The model under review builds one solid part; all positions refer to its coordinate system, in mm. A direction names the side the tool comes from. Round coordinates to 2 decimals unless told otherwise and drop trailing zeros. Write each loop counter-clockwise with the first axis right and the second up, starting at its lowest first coordinate (ties: lowest second). Pieces come first, ordered by that corner, then holes. Notation, with made-up numbers: (82, -16) -> (139, -16) arc R29 cw to (139, 4) -> close; hole circle Ø9 at (50.25, 41). An arc over 180 degrees is marked (long way). Answer as a JSON object with one key per item and string values. Group by question number.
1) Machinability: for faces 5 (the flat face through (-9.605, -0.089, 50.386)), 6 (the flat face through (-41.67, -0.09, -44.02)), 7 (the flat face through (-1, 0, 9.919)), 8 (the flat face through (101.346, 0, -27)), which of the approach directions +Z, -Z, +X, -X, +Y, -Y give a long, thin tool a straight path to every point of the face, cutting with its end or side? Answer none if there is none.
2) We need section A-A, the plane x = -20. Write out the cut boundary in (y, z).
3) We need section D-D, the plane x = 56. Write out the cut boundary in (y, z), then the cut area to 3 significant figures.
4) To check wall thickness, follow probe 1 along Z at (x, y) = (-4.5, -4.25); probe 2 along Z at (x, y) = (28, -4.75); probe 3 along X at (y, z) = (4.5, 41). State the ranges of each line that lie inside material, in increasing order. Write a range as [from, to].
5) Insertion check: pin 1 Ø2 at (x, y) = (-40, 4.5) entering from -Z; pin 2 Ø4 at (x, y) = (-4, -1.5) entering from -Z; pin 3 Ø6.5 at (x, y) = (91, -1.5) entering from +Z. Each pin has a flat end and moves straight along its axis. Give the tip position at first contact, or say it passes through.
6) We need section C-C, the plane z = -14. Write out the cut boundary in (x, y), then the cut area to 3 significant figures.
7) Mouldability with a two-part tool opening along Z and no side actions: class faces 1 (the flat face through (89, 0, -16.37)), 2 (the flat face through (-1, -6.35, -18)), 3 (the flat face through (9.697, -0.089, 50.731)), 4 (the flat face through (-75.946, 0, -7)) as pulls with the +Z half, pulls with the -Z half, needs draft (parallel to the pull), parting line crosses it, or undercut.
from build123d import *

# Parameters (mm, degrees)
F1_DEPTH = 6.35
F2_SIZE  = 12.446


with BuildPart() as f1:
    # F0 (on Front) → F1 (new body, symmetric)
    with BuildSketch(Plane.XZ):
        with BuildLine():
            Line((6.35, 38.239533), (0, 38.239533))
            Line((0, 38.239533), (-6.35, 38.239533))
            Line((-6.35, 38.239533), (-12.951732, 62.877533))
            Line((-12.951732, 62.877533), (-28.495513, 62.877533))
            ThreePointArc((-28.495513, 62.877533), (-39.577525, 59.32242), (-46.523284, 49.983992))
            ThreePointArc((-46.523284, 49.983992), (-55.553194, 36.446133), (-70.104, 29.160052))
            Line((-70.104, 29.160052), (-91.232227, 24.765415))
            ThreePointArc((-91.232227, 24.765415), (-98.498286, 20.345425), (-101.346, 12.331533))
            Line((-101.346, 12.331533), (-101.346, 2.679533))
            Line((-101.346, 2.679533), (-75.946, 2.679533))
            Line((-75.946, 2.679533), (-75.946, -16.370467))
            Line((-75.946, -16.370467), (-101.346, -16.370467))
            Line((-101.346, -16.370467), (-101.346, -50.152467))
            Line((-101.346, -50.152467), (-45.212, -50.152467))
            Line((-45.212, -50.152467), (-38.026299, -37.706467))
            Line((-38.026299, -37.706467), (0, -37.706467))
            Line((0, -37.706467), (38.026299, -37.706467))
            Line((38.026299, -37.706467), (45.212, -50.152467))
            Line((45.212, -50.152467), (101.346, -50.152467))
            Line((101.346, -50.152467), (101.346, -16.370467))
            Line((101.346, -16.370467), (75.946, -16.370467))
            Line((75.946, -16.370467), (75.946, 2.679533))
            Line((75.946, 2.679533), (101.346, 2.679533))
            Line((101.346, 2.679533), (101.346, 12.331533))
            ThreePointArc((101.346, 12.331533), (98.498286, 20.345425), (91.232227, 24.765415))
            Line((91.232227, 24.765415), (70.104, 29.160052))
            ThreePointArc((70.104, 29.160052), (55.553194, 36.446133), (46.523284, 49.983992))
            ThreePointArc((46.523284, 49.983992), (39.577525, 59.32242), (28.495513, 62.877533))
            Line((28.495513, 62.877533), (12.951732, 62.877533))
            Line((12.951732, 62.877533), (6.35, 38.239533))
        make_face()
        with BuildLine():
            ThreePointArc((-33.38948, -9.131467), (-42.91448, 0.393533), (-33.38948, 9.918533))
            Line((-33.38948, 9.918533), (31.75, 9.918533))
            ThreePointArc((31.75, 9.918533), (41.275, 0.393533), (31.75, -9.131467))
            Line((31.75, -9.131467), (-33.38948, -9.131467))
        make_face(mode=Mode.SUBTRACT)
    extrude(amount=F1_DEPTH, both=True)

    # F2
    f2_edges = [f1.edges().sort_by_distance(p)[0] for p in [
        (-101.346, 0, -50.152467),
        (101.346, 0, -50.152467),
    ]]
    chamfer(f2_edges, length=F2_SIZE)


solid = f1.part
Here are the results:
{
 "1": {"face 5": "+Z, +Y, -Y", "face 6": "-Z, +Y, -Y", "face 7": "+Y, -Y", "face 8": "+Z, -Z, +X, +Y, -Y"},
 "2": {"outline": "(-6.35, -37.71) -> (6.35, -37.71) -> (6.35, -9.13) -> (-6.35, -9.13) -> close; (-6.35, 9.92) -> (6.35, 9.92) -> (6.35, 62.88) -> (-6.35, 62.88) -> close"},
 "3": {"outline": "(-6.35, -50.15) -> (6.35, -50.15) -> (6.35, 36.06) -> (-6.35, 36.06) -> close", "area": "1,090 mm^2"},
 "4": {"probe 1": "z = [-37.71, -9.13], [9.92, 38.24]", "probe 2": "z = [-37.71, -9.13], [9.92, 62.88]", "probe 3": "x = [-51.32, -7.09], [7.09, 51.32]"},
 "5": {"pin 1": "stops at z = -42.86", "pin 2": "stops at z = -37.71", "pin 3": "stops at z = 25.49"},
 "6": {"outline": "(-75.95, -6.35) -> (75.95, -6.35) -> (75.95, 6.35) -> (-75.95, 6.35) -> close", "area": "1,930 mm^2"},
 "7": {"face 1": "undercut", "face 2": "needs draft", "face 3": "pulls with the +Z half", "face 4": "undercut"}
}
